Source: CAD feature listing. Evaluate the final solid. Frame: model axes, mm. Coordinates: 2 decimals unless noted, no trailing zeros. Loops run counter-clockwise (first coordinate to the right, second up) from the corner with the lowest first, then second, coordinate; pieces in that order, holes last. Notation, with made-up numbers: (-35.5, 0.25) -> (3.5, 0.25) arc R25 cw to (3.5, 26.25) -> close; hole circle Ø3 at (84.5, 51). An arc over 180 degrees is marked (long way). Answer as a JSON object with one key per item and string values. Group by question number.
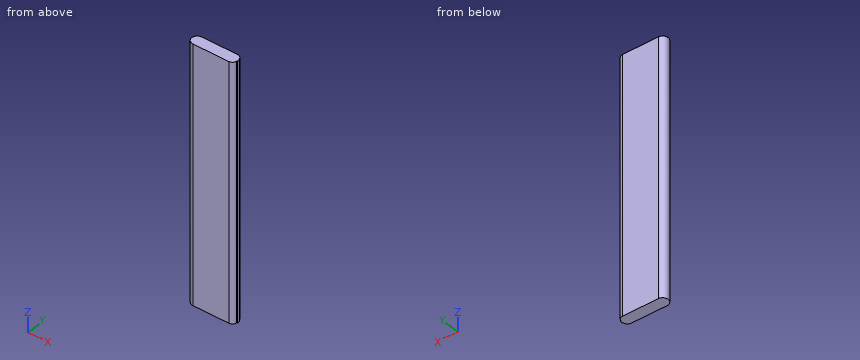
from build123d import *

# Parameters (mm, degrees)
BOSS_EXTRUDE1_DEPTH = 82.5


with BuildPart() as part:
    # Sketch1 → Boss-Extrude1 (new, symmetric)
    with BuildSketch(Plane.XY):
        with BuildLine():
            Line((-11.25, 3.5), (11.25, 3.5))
            ThreePointArc((11.25, 3.5), (13.194543648, 2.694543648), (14, 0.75))
            Line((14, 0.75), (14.5, 0.75))
            Line((14.5, 0.75), (14.5, -0.75))
            Line((14.5, -0.75), (14, -0.75))
            ThreePointArc((14, -0.75), (13.194543648, -2.694543648), (11.25, -3.5))
            Line((11.25, -3.5), (-11.25, -3.5))
            ThreePointArc((-11.25, -3.5), (-14.75, 0), (-11.25, 3.5))
        make_face()
    extrude(amount=BOSS_EXTRUDE1_DEPTH, both=True)


solid = part.part
1. Ray query, L1, parallel to X at y = 0.25, z = -29.5; L2, parallel to X at y = -2.5, z = 71.5; L3, parallel to Y at x = 13, z = -1. Return the intervals inside material, ascending.
2. Section query A-A on z = -9.5. Return loops of the section in (x, y), then the cut area to 3 significant figures.
3. Section query B-B on y = -2.25. Return loops of the section in (x, z).
Solved:
{
 "1": {"L1": "-14.74 to 14.5", "L2": "-13.7 to 13.37", "L3": "-2.87 to 2.87"},
 "2": {"outline": "(-11.25, -3.5) -> (11.25, -3.5) arc R2.75 ccw to (14, -0.75) -> (14.5, -0.75) -> (14.5, 0.75) -> (14, 0.75) arc R2.75 ccw to (11.25, 3.5) -> (-11.25, 3.5) arc R3.5 ccw to start", "area": "193 mm^2"},
 "3": {"outline": "(-13.93, -82.5) -> (13.55, -82.5) -> (13.55, 82.5) -> (-13.93, 82.5) -> close"}
}
